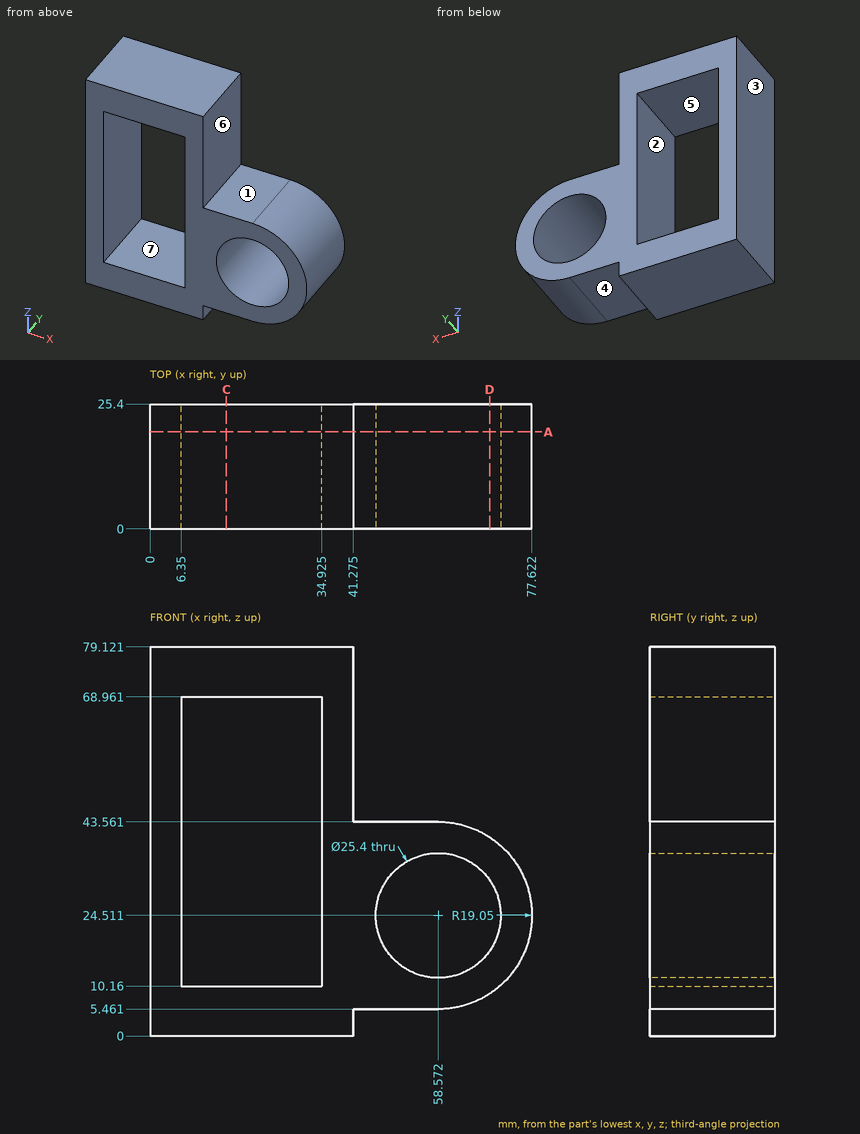
Check sheet for the drawn part. Datum: minimum x, y, z corner. Units: mm. A direction names the side the tool comes from. Give positions to 0.01 mm unless a question says otherwise; leave off trailing zeros. Write each loop counter-clockwise with the first axis right and the second up, starting at its lowest first coordinate (ties: lowest second). Pieces come first, ordered by that corner, then holes. Notation, with made-up numbers: M -31.75,43.5 L 23.25,43.5 A12 ccw 23.25,58.5 Z; hole C 29,70 d7. An arc over 180 degrees is marked long. Write item = value, one per line.
(1) Sectioned sample at A-A (y = 19.75). Give the number of separate pieces and of enclosed holes in the cut face, then the cut area to 3 significant figures.
Found:
separate_pieces = 1
enclosed_holes = 2
area = 2,310 mm2
(2) Material ranges on line 1 (Z direction, x = 31, y = 22.25); line 2 (Z direction, x = 69, y = 8) (1 decimal); line 3 (X direction, y = 8.5, z = 69.5) (1 decimal), recorded low to high.
Found:
line_1 = 0 to 10.16, 68.96 to 79.12
line_2 = 8.6 to 17.3, 31.8 to 40.5
line_3 = 0 to 41.3
(3) Sectioned sample at D-D (x = 69). Record the cut outline in (y, z), then the cut area to 3 significant figures.
Found:
outline = M 0,8.57 L 25.4,8.57 L 25.4,17.26 L 0,17.26 Z; M 0,31.76 L 25.4,31.76 L 25.4,40.45 L 0,40.45 Z
area = 442 mm2
(4) Go/stop test with flat-tipped pins: pin 1 Ø8 at (x, y) = (53, 13.5) entering from -Z; pin 2 Ø12.5 at (x, y) = (22, 19) entering from -Z; pin 3 Ø6 at (x, y) = (62, 9) entering from +Z; pin 4 Ø20.5 at (x, z) = (58.57, 24.51) entering from +Y. Record where each tip stops, or that it passes through.
Found:
pin_1 = 5.46
pin_2 = 0
pin_3 = 43.56
pin_4 = through
(5) Sectioned sample at C-C (x = 15.5). Record the cut outline in (y, z).
Found:
outline = M 0,0 L 25.4,0 L 25.4,10.16 L 0,10.16 Z; M 0,68.96 L 25.4,68.96 L 25.4,79.12 L 0,79.12 Z
(6) Access from +Z, -Z, +X, -X, +Y, -Y to the whole of each face (thin tool, end or side, straight path). Record for the marked faces 1, 2 and 3.
Found:
face_1 = +Z, +X, +Y, -Y
face_2 = +Y, -Y
face_3 = +Z, -Z, -X, +Y, -Y
(7) Draft check along X on the marked faces 4, 5, 6 and 7. Enter one of: released by +X, released by -X, zero draft, split by the parting line, or undercut.
Found:
face_4 = zero draft
face_5 = undercut
face_6 = released by +X
face_7 = undercut
